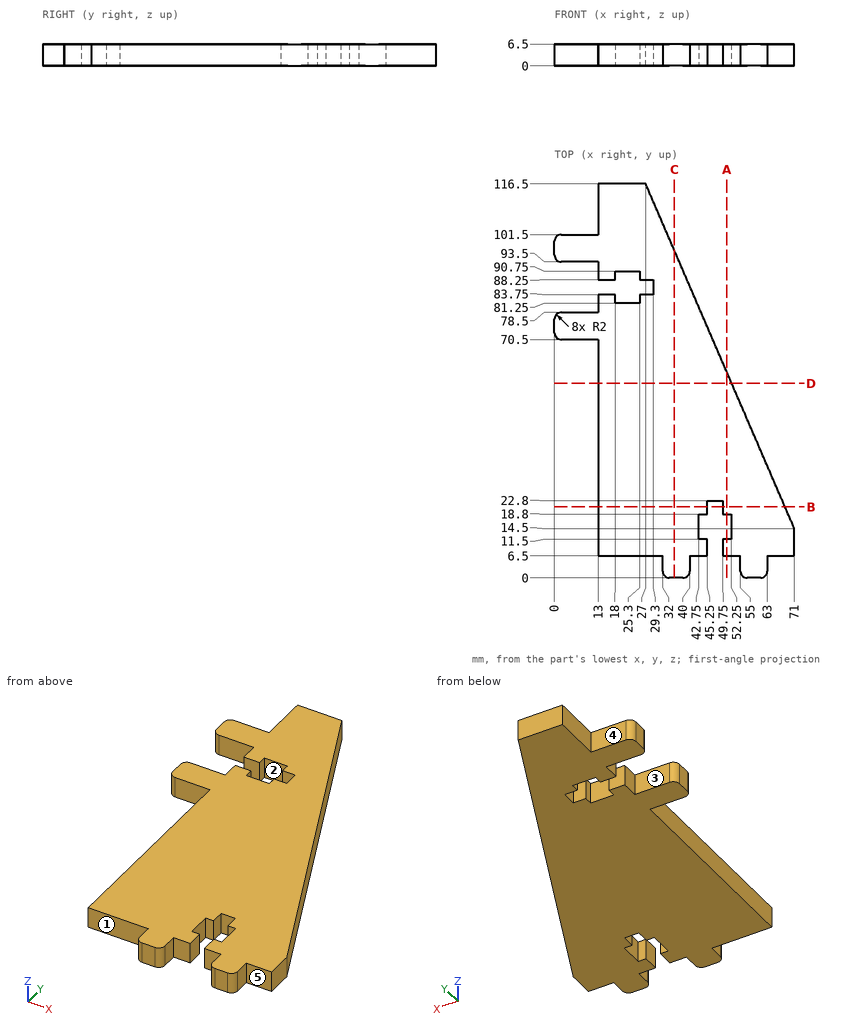
Source: three-view drawing plus pictorial views. Frame: mm from the lowest corner of the part. A direction names the side the tool comes from. Coordinates: 2 decimals unless noted, no trailing zeros. Order: outer loops, then holes, each group sorted by start corner. A loop starts at its lowest first (then second) coordinate and runs counter-clockwise, first axis right, second up.
1) First-contact query: P1, Ø2, axis at x = 22, z = 4, coming from the -Y side; P2, Ø3, axis at y = 51, z = 5, coming from the -X side; P3, Ø3, axis at x = 37, y = 20.5, coming from the -Z side; P4, Ø2, axis at y = 83, z = 3, coming from the +X side. Flat tips, straight axial feed; report the tip coordinate or a pass-through.
Result sheet:
P1: stops at y = 6.5
P2: stops at x = 13
P3: stops at z = 0
P4: stops at x = 41.88
2) Ray query, probe 1 along Y at (x, z) = (22, 3); probe 2 along Y at (x, z) = (15, 2.5); probe 3 along Y at (x, z) = (37.5, 4.5). Return the intervals inside material, ascending.
Result sheet:
probe 1: y = 6.5 to 81.25, 90.75 to 116.5
probe 2: y = 6.5 to 83.75, 88.25 to 116.5
probe 3: y = 0 to 92.16
3) Section A-A (x = 51). Return loops of the section in (y, z).
Result sheet:
outline: (6.5, 0) - (11.5, 0) - (11.5, 6.5) - (6.5, 6.5) - close; (18.8, 0) - (60.86, 0) - (60.86, 6.5) - (18.8, 6.5) - close
4) Set-up query: the marked faces 1, 2, 3, 4 and 5. Return all of +Z, -Z, +X, -X, +Y, -Y with unobstructed straight access to the full face (end or side cutting, diameter ignored); none if empty.
Result sheet:
face 1: +Z, -Z, -X, -Y
face 2: +Z, -Z
face 3: +Z, -Z, -X
face 4: +Z, -Z, -X, +Y
face 5: +Z, -Z, +X, -Y
5) Section B-B (y = 21). Return loops of the section in (x, z).
Result sheet:
outline: (13, 0) - (45.25, 0) - (45.25, 6.5) - (13, 6.5) - close; (49.75, 0) - (68.2, 0) - (68.2, 6.5) - (49.75, 6.5) - close
6) Section C-C (x = 35.5). Return loops of the section in (y, z).
Result sheet:
outline: (0, 0) - (96.8, 0) - (96.8, 6.5) - (0, 6.5) - close
7) Section D-D (y = 57.5). Return loops of the section in (x, z), then the cut area to 3 significant figures.
Result sheet:
outline: (13, 0) - (52.45, 0) - (52.45, 6.5) - (13, 6.5) - close
area: 256 mm2
